Source: CAD feature listing. Evaluate the final solid. Frame: model axes, mm. Face numbers are marked on the shaded views. A direction names the side the tool comes from. Coordinates: 2 decimals unless noted, no trailing zeros. Order: outer loops, then holes, each group sorted by start corner. A loop starts at its lowest first (then second) coordinate and runs counter-clockwise, first axis right, second up. Notation, with made-up numbers: (10, 71) - (49, 71) arc R22 ccw to (49, 98) - close; hole circle Ø3 at (-19, 8.25). An arc over 180 degrees is marked (long way). One line per question, with ' | ' between items.
from build123d import *

# Parameters (mm, degrees)
SKETCH1_R           = 8.5
BOSS_EXTRUDE1_DEPTH = 1.5
SKETCH1_4_R         = 15
SKETCH1_4_R_2       = 8.5
BOSS_EXTRUDE2_DEPTH = 12.5
CUT_EXTRUDE1_START  = 2
SKETCH2_W           = 16.8
SKETCH2_H           = 15
CUT_EXTRUDE1_DEPTH  = 24.416530054
FILLET1_R           = 3
SKETCH3_R           = 3.15
CUT_EXTRUDE2_DEPTH  = 26.102558411
FILLET3_SIZE        = 1.5
BOSS_EXTRUDE3_DEPTH = 1
CHAMFER1_SIZE       = 2


with BuildPart() as part:
    # Sketch1 → Boss-Extrude1 (new body)
    with BuildSketch(Plane.XY):
        Circle(SKETCH1_R)
    extrude(amount=BOSS_EXTRUDE1_DEPTH)

    # Sketch1<4> → Boss-Extrude2 (add)
    # profile 1 of 7: a face of its own
    with BuildSketch(Plane.XY):
        Circle(SKETCH1_4_R)
        with Locations(Location((0, 0, 0), (0, 0, 180))):
            Circle(SKETCH1_4_R_2, mode=Mode.SUBTRACT)
    # profile 2 of 7: a face of its own
    with BuildSketch(Plane.XY):
        with BuildLine():
            Line((12.990381063, 7.499999988), (8.660254038, 15))
            Line((8.660254038, 15), (-1.6e-08, 15))
            ThreePointArc((-1.6e-08, 15), (7.499999999, 12.990381058), (12.990381063, 7.499999988))
        make_face()
    # profile 3 of 7: a face of its own
    with BuildSketch(Plane.XY):
        with BuildLine():
            ThreePointArc((-12.99038099, 7.500000116), (-7.499999949, 12.990381086), (-1.6e-08, 15))
            Line((-1.6e-08, 15), (-8.660254038, 15))
            Line((-8.660254038, 15), (-12.99038099, 7.500000116))
        make_face()
    # profile 4 of 7: a face of its own
    with BuildSketch(Plane.XY):
        with BuildLine():
            ThreePointArc((-12.990380876, -7.500000313), (-15, -1.14e-07), (-12.99038099, 7.500000116))
            Line((-12.99038099, 7.500000116), (-17.320508076, 0))
            Line((-17.320508076, 0), (-12.990380876, -7.500000313))
        make_face()
    # profile 5 of 7: a face of its own
    with BuildSketch(Plane.XY):
        with BuildLine():
            Line((17.320508076, 0), (12.990381063, 7.499999988))
            ThreePointArc((12.990381063, 7.499999988), (14.488887396, 3.88228567), (15, 0))
            ThreePointArc((15, 0), (14.488887391, -3.88228569), (12.990381043, -7.500000024))
            Line((12.990381043, -7.500000024), (17.320508076, 0))
        make_face()
    # profile 6 of 7: a face of its own
    with BuildSketch(Plane.XY):
        with BuildLine():
            Line((8.660254038, -15), (12.990381043, -7.500000024))
            ThreePointArc((12.990381043, -7.500000024), (7.499999988, -12.990381064), (0, -15))
            Line((0, -15), (8.660254038, -15))
        make_face()
    # profile 7 of 7: a face of its own
    with BuildSketch(Plane.XY):
        with BuildLine():
            ThreePointArc((0, -15), (-7.499999843, -12.990381147), (-12.990380876, -7.500000313))
            Line((-12.990380876, -7.500000313), (-8.660254038, -15))
            Line((-8.660254038, -15), (0, -15))
        make_face()
    extrude(amount=BOSS_EXTRUDE2_DEPTH)

    # Sketch2 → Cut-Extrude1 (cut, through all)
    with BuildSketch(Plane.XY.offset(1.5).offset(CUT_EXTRUDE1_START)):
        with Locations((0, -7.5)):
            Rectangle(SKETCH2_W, SKETCH2_H)
    extrude(amount=CUT_EXTRUDE1_DEPTH, mode=Mode.SUBTRACT)

    # Fillet1
    fillet1_edges = [part.edges().sort_by_distance(p)[0] for p in [
        (17.320508076, 0, 6.25),
        (8.660254038, 15, 6.25),
        (-8.660254038, 15, 6.25),
        (-17.320508076, 0, 6.25),
    ]]
    fillet(fillet1_edges, radius=FILLET1_R)

    # Sketch3 → Cut-Extrude2 (cut, through all)
    with BuildSketch(Plane.XY.offset(1.5)):
        Circle(SKETCH3_R)
    extrude(amount=-CUT_EXTRUDE2_DEPTH, mode=Mode.SUBTRACT)

    # Fillet3
    fillet3_edges = [part.edges().sort_by_distance(p)[0] for p in [
        (-12.557368355, -8.25, 0),
        (12.990381057, 7.5, 0),
        (-12.990381057, 7.5, 0),
        (0, 15, 0),
        (16.856406461, 0, 0),
        (8.42820323, 14.598076211, 0),
        (-8.42820323, 14.598076211, 0),
        (-16.856406461, 0, 0),
        (0, -15, 0),
        (12.557368355, -8.25, 0),
    ]]
    chamfer(fillet3_edges, length=FILLET3_SIZE)

    # Sketch5 → Boss-Extrude3 (add)
    with BuildSketch(Plane.XY.offset(12.5)):
        with BuildLine():
            Line((-10.392304845, -16), (-8.660254038, -15))
            Line((-8.660254038, -15), (-16.454482672, -1.5))
            ThreePointArc((-16.454482672, -1.5), (-16.856406461, 0), (-16.454482672, 1.5))
            Line((-16.454482672, 1.5), (-9.526279442, 13.5))
            ThreePointArc((-9.526279442, 13.5), (-8.42820323, 14.598076211), (-6.92820323, 15))
            Line((-6.92820323, 15), (6.92820323, 15))
            ThreePointArc((6.92820323, 15), (8.42820323, 14.598076211), (9.526279442, 13.5))
            Line((9.526279442, 13.5), (16.454482672, 1.5))
            ThreePointArc((16.454482672, 1.5), (16.856406461, 0), (16.454482672, -1.5))
            Line((16.454482672, -1.5), (8.660254038, -15))
            Line((8.660254038, -15), (10.392304845, -16))
            Line((10.392304845, -16), (18.186533479, -2.5))
            ThreePointArc((18.186533479, -2.5), (18.856406461, 0), (18.186533479, 2.5))
            Line((18.186533479, 2.5), (11.258330249, 14.5))
            ThreePointArc((11.258330249, 14.5), (9.42820323, 16.330127019), (6.92820323, 17))
            Line((6.92820323, 17), (-6.92820323, 17))
            ThreePointArc((-6.92820323, 17), (-9.42820323, 16.330127019), (-11.258330249, 14.5))
            Line((-11.258330249, 14.5), (-18.186533479, 2.5))
            ThreePointArc((-18.186533479, 2.5), (-18.856406461, 0), (-18.186533479, -2.5))
            Line((-18.186533479, -2.5), (-10.392304845, -16))
        make_face()
    extrude(amount=-BOSS_EXTRUDE3_DEPTH)

    # Chamfer1
    chamfer1_edges = [part.edges().sort_by_distance(p)[0] for p in [
        (12.557368355, -8.25, 11.5),
        (16.856406461, 0, 11.5),
        (12.990381057, 7.5, 11.5),
        (8.42820323, 14.598076211, 11.5),
        (0, 15, 11.5),
        (-8.42820323, 14.598076211, 11.5),
        (-12.990381057, 7.5, 11.5),
        (-16.856406461, 0, 11.5),
        (-12.557368355, -8.25, 11.5),
    ]]
    chamfer(chamfer1_edges, length=CHAMFER1_SIZE - 0.0001)  # a hair under: the kernel refuses the full size


solid = part.part
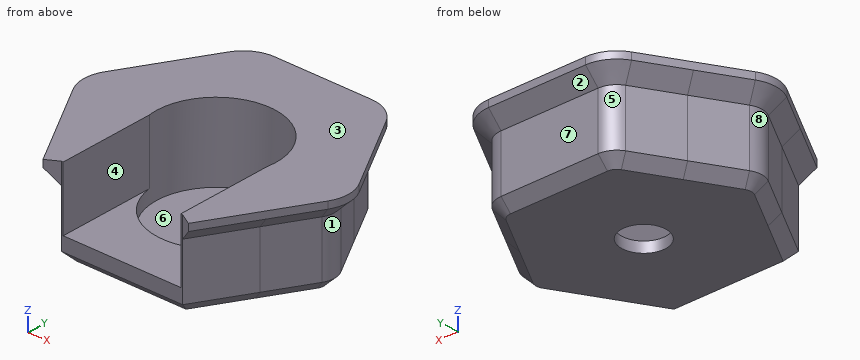
(1) Pull-direction query (Z, two-part tool) for the marked faces 1, 2 and 3; classes: pulls with the +Z half, pulls with the -Z half, needs draft (parallel to the pull), parting line crosses it, or undercut.
Taken from the geometry:
face 1: needs draft | face 2: pulls with the -Z half | face 3: pulls with the +Z half
(2) Pin query (flat end, axial travel): P1, Ø11, axis at x = 0, y = -8.5, coming from the +Z side; P2, Ø3, axis at y = 9.5, z = 8, coming from the +X side; P3, Ø5, axis at x = -1, y = -3.5, coming from the +Z side. Return the tip coordinate at first contact, or that it passes through.
Taken from the geometry:
P1: stops at z = 3.5 | P2: stops at x = 12.7 | P3: stops at z = 1.5
(3) Material intervals for L1, parallel to Z at x = -7, y = -10.5; L2, parallel to X at y = -14, z = 11.5; L3, parallel to Y at x = 6, z = 1.75, sorted ascending. Write a range as from..to.
Taken from the geometry:
L1: z = 0..3.5 | L2: x = -11.55..-8.4, 8.4..11.55 | L3: y = -15..-6.02, 6.02..15
(4) Set-up query: the marked faces 4, 5, 6, 7 and 8. Return all of +Z, -Z, +X, -X, +Y, -Y with unobstructed straight access to the full face (end or side cutting, diameter ignored); none if empty.
Taken from the geometry:
face 4: +Z, -Y | face 5: -Z, -X, +Y | face 6: +Z | face 7: -Z, +X, -X, +Y | face 8: -Z, -X
(5) Cut plane B-B (z = 9). Return the cut outline in (x, y), and give its area (3 significant figures).
Taken from the geometry:
outline: (-16.45, -1.5) - (-8.66, -15) - (-8.4, -15) - (-8.4, -1.3) arc R8.5 cw (long way) to (8.4, -1.3) - (8.4, -15) - (8.66, -15) - (16.45, -1.5) arc R3 ccw to (16.45, 1.5) - (9.53, 13.5) arc R3 ccw to (6.93, 15) - (-6.93, 15) arc R3 ccw to (-9.53, 13.5) - (-16.45, 1.5) arc R3 ccw to start | area: 412 mm²
(6) Cut plane C-C (z = 1). Return the cut outline in (x, y).
Taken from the geometry:
outline: (-16.02, -1.25) - (-8.37, -14.5) - (8.37, -14.5) - (16.02, -1.25) arc R2.5 ccw to (16.02, 1.25) - (9.09, 13.25) arc R2.5 ccw to (6.93, 14.5) - (-6.93, 14.5) arc R2.5 ccw to (-9.09, 13.25) - (-16.02, 1.25) arc R2.5 ccw to start; hole circle Ø6.3 at (0, 0)
